Check sheet for the drawn part. Datum: minimum x, y, z corner. Units: mm. Give positions to 0.01 mm unless a question says otherwise; leave off trailing zeros. Loops run counter-clockwise (first coordinate to the right, second up) from the corner with the lowest first, then second, coordinate; pieces in that order, holes last. Notation, with made-up numbers: (8, 67) - (12, 67) arc R18 ccw to (12, 85) - close; hole circle Ø2 at (8.25, -11.75). An arc over 180 degrees is marked (long way). Use one line per item in the form item = value.
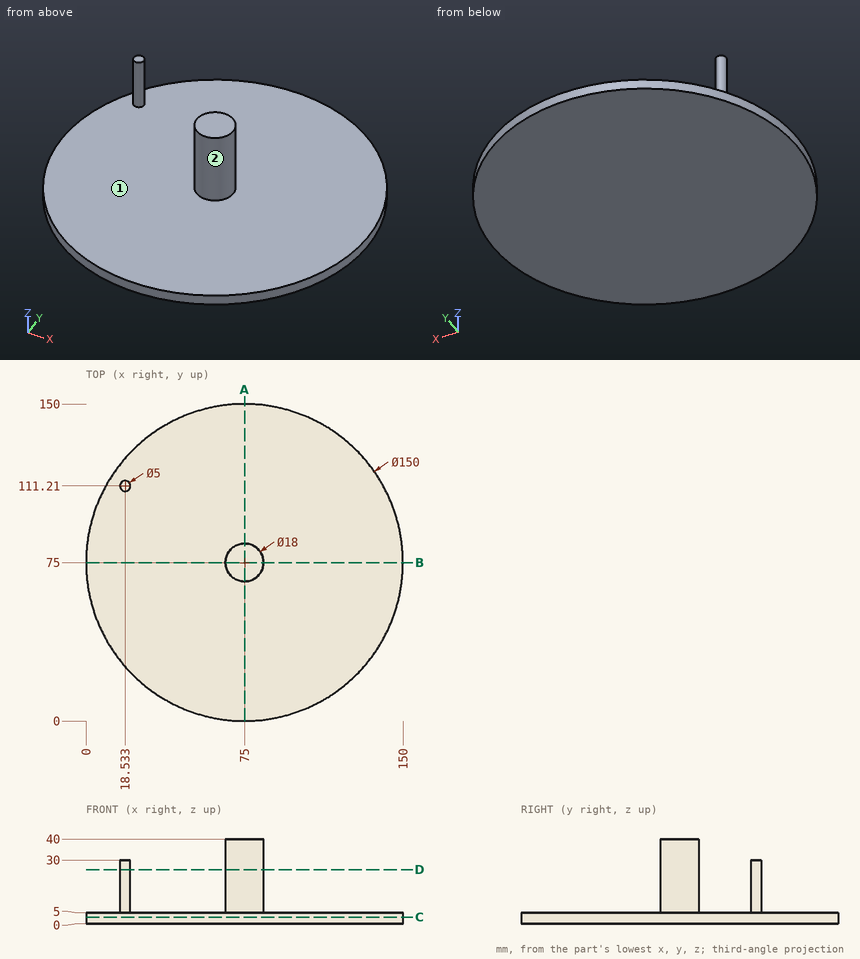
Item 1: Thickness scan on L1, parallel to Z at x = 123, y = 84.5; L2, parallel to X at y = 17.5, z = 3; L3, parallel to Y at x = 75, z = 6.5. Record the ranges inside material, lowest first.
Answer block:
L1 = 0 to 5
L2 = 26.85 to 123.15
L3 = 66 to 84
Item 2: Section check A-A on x = 75. Record the boundary of the cut face in (y, z), then the cut area to 3 significant figures.
Answer block:
outline = (0, 0) - (150, 0) - (150, 5) - (84, 5) - (84, 40) - (66, 40) - (66, 5) - (0, 5) - close
area = 1,380 mm2
Item 3: Section check D-D on z = 25.5. Record the boundary of the cut face in (x, y).
Answer block:
outline = circle Ø5 at (18.53, 111.21); circle Ø18 at (75, 75)
Item 4: Gauge pin test, flat ends, axial feed: P1, Ø10, axis at y = 83.5, z = 27.5, coming from the +X side; P2, Ø4, axis at x = 63.5, y = 49.5, coming from the +Z side; P3, Ø4, axis at x = 17.5, y = 110.5, coming from the +Z side. Record the tip position at first contact, or that the pin passes through.
Answer block:
P1 = 83.29
P2 = 5
P3 = 30
Item 5: Mould release check, pull along Y, two halves, no side actions. Record for the marked faces 1 and 2: released by +Y, released by -Y, zero draft, split by the parting line, or undercut.
Answer block:
face_1 = zero draft
face_2 = split by the parting line
Item 6: Section check C-C on z = 3. Record the boundary of the cut face in (x, y).
Answer block:
outline = circle Ø150 at (75, 75)
